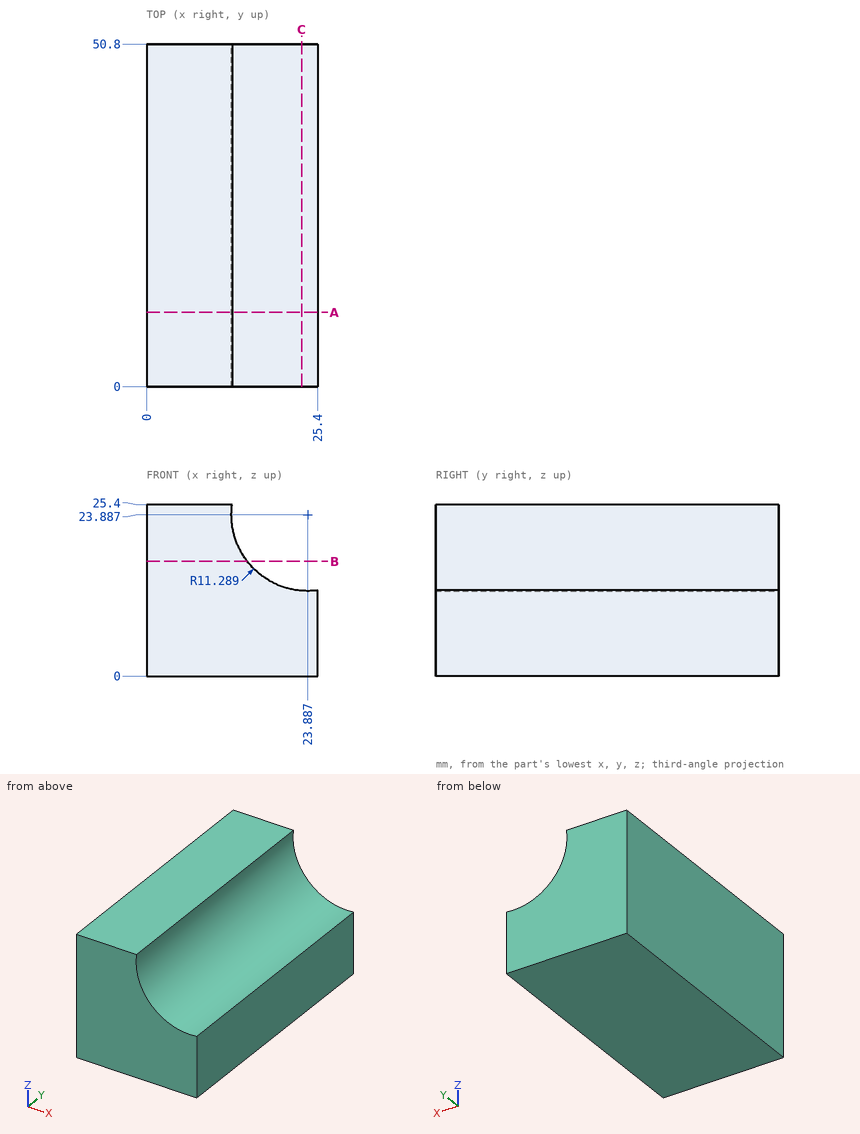
The drawing under review shows one solid part. Ordinate dimensions are in mm from its lowest x, y, z. Coordinates: 2 decimals unless noted, no trailing zeros. Write each loop counter-clockwise with the first axis right and the second up, starting at its lowest first coordinate (ties: lowest second). Pieces come first, ordered by that corner, then holes. Notation, with made-up numbers: (-3.75, 65.5) -> (23.25, 65.5) arc R21 ccw to (23.25, 80.5) -> close; hole circle Ø11 at (-32, 27.5). An arc over 180 degrees is marked (long way). Write each question's results on one line, items separated by ' | '. Start each with the question number.
1) Consider section C-C (x = 23). Write out the cut boundary in (y, z), plus the area to 3 significant figures.
2) Wall thickness on L1, parallel to X at y = 29, z = 24; L2, parallel to X at y = 17.5, z = 22: over which ranges is each line inside the solid? List them lowest first. Write a range as [from, to].
3) Consider section A-A (y = 11). Write out the cut boundary in (x, z).
4) Insertion check: pin 1 (5 mm diameter, centred on y = 12, z = 19, fed in from +X). The pin has a flat end and moves straight along its axis. Give the tip position at first contact, or say it passes through.
5) Consider section B-B (z = 17). Write out the cut boundary in (x, y).
Geometry says:
1) outline: (0, 0) -> (50.8, 0) -> (50.8, 12.63) -> (0, 12.63) -> close | area: 642 mm^2
2) L1: [0, 12.6] | L2: [0, 12.76]
3) outline: (0, 0) -> (25.4, 0) -> (25.4, 12.7) arc R11.29 cw to (12.7, 25.4) -> (0, 25.4) -> close
4) pin 1: x = 15.35
5) outline: (0, 0) -> (14.94, 0) -> (14.94, 50.8) -> (0, 50.8) -> close
